Print and shaded views of the part. All mm, measured from the part's lowest x, y and z. A direction names the side the tool comes from. Round coordinates to 2 decimals unless told otherwise and drop trailing zeros. Order: outer loops, then holes, each group sorted by start corner. A loop starts at its lowest first (then second) coordinate and runs counter-clockwise, first axis right, second up. Notation, with made-up numbers: (75, 11.25) - (107, 11.25) arc R17 cw to (107, 38.25) - close; hole circle Ø2 at (-24, -25). An arc over 180 degrees is marked (long way). Write item = value, one per line.
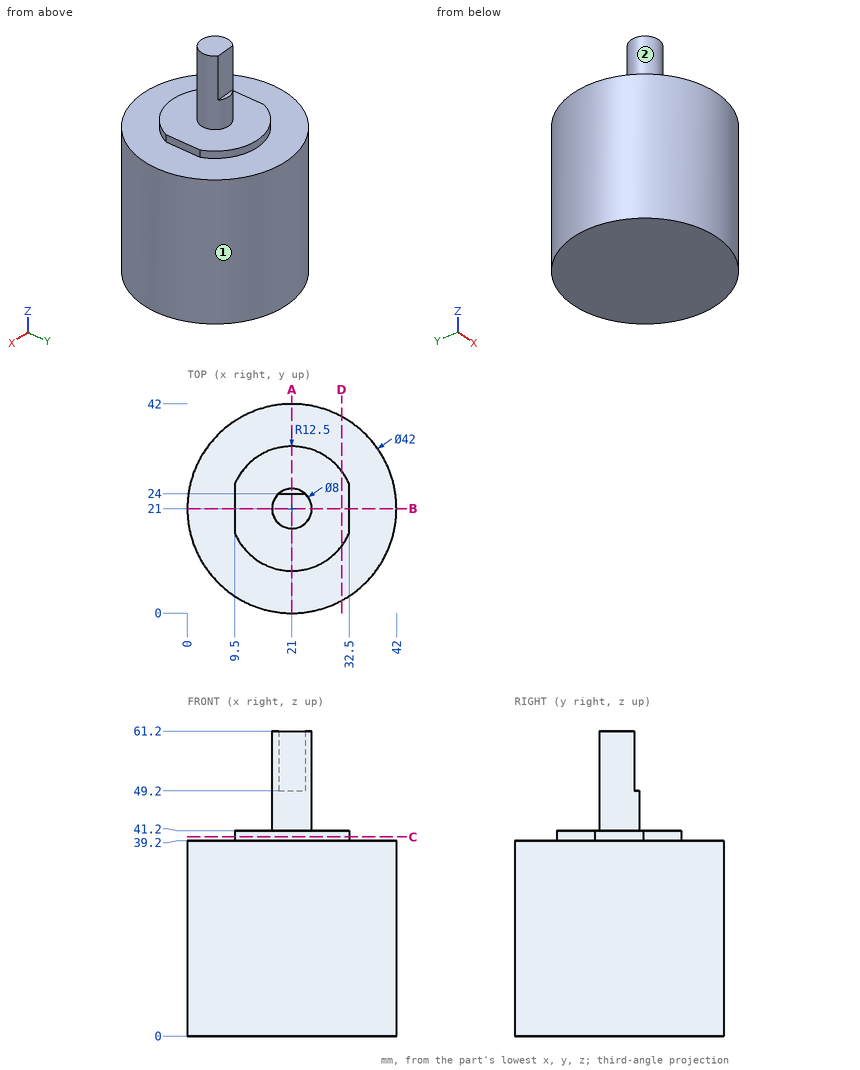
(1) Band-saw the part on A-A on x = 21. List the corners of the cut face in (y, z), plus the area to 3 significant figures.
Solved:
outline = (0, 0) - (42, 0) - (42, 39.2) - (33.5, 39.2) - (33.5, 41.2) - (25, 41.2) - (25, 49.2) - (24, 49.2) - (24, 61.2) - (17, 61.2) - (17, 41.2) - (8.5, 41.2) - (8.5, 39.2) - (0, 39.2) - close
area = 1,840 mm²
(2) Band-saw the part on B-B on y = 21. List the corners of the cut face in (x, z).
Solved:
outline = (0, 0) - (42, 0) - (42, 39.2) - (32.5, 39.2) - (32.5, 41.2) - (25, 41.2) - (25, 61.2) - (17, 61.2) - (17, 41.2) - (9.5, 41.2) - (9.5, 39.2) - (0, 39.2) - close
(3) Band-saw the part on D-D on x = 31. List the corners of the cut face in (y, z).
Solved:
outline = (2.53, 0) - (39.47, 0) - (39.47, 39.2) - (28.5, 39.2) - (28.5, 41.2) - (13.5, 41.2) - (13.5, 39.2) - (2.53, 39.2) - close
(4) Probe line 1 along Z through (x, y) = (10.5, 33); line 2 along Z through (x, y) = (12.5, 28.5); line 3 along X through (y, z) = (17.5, 8.5). List the from-to ranges inside material, lowest first.
Solved:
line_1 = 0 to 39.2
line_2 = 0 to 41.2
line_3 = 0.29 to 41.71
(5) Band-saw the part on C-C on z = 40. List the corners of the cut face in (x, y).
Solved:
outline = (9.5, 16.1) arc R12.5 ccw to (32.5, 16.1) - (32.5, 25.9) arc R12.5 ccw to (9.5, 25.9) - close
(6) Drop flat-ended pins along their axis: pin 1 (6 mm diameter, centred on x = 29, y = 23, fed in from +Z); pin 2 (0.5 mm diameter, centred on x = 21, y = 24.5, fed in from +Z); pin 3 (12 mm diameter, centred on y = 10.5, z = 54, fed in from +X) (3 decimals); pin 4 (6 mm diameter, centred on y = 25, z = 32, fed in from -X). Give the stop position or say it passes through.
Solved:
pin_1 = 41.2
pin_2 = 49.2
pin_3 = through
pin_4 = 0.02
(7) Tool access for the marked faces 1 and 2: list every direction of +Z, -Z, +X, -X, +Y, -Y with a clear straight run to the whole face (end or side of a thin tool).
Solved:
face_1 = +Z, -Z
face_2 = +Z
